```python
from build123d import *

# Parameters (mm, degrees)
SKETCH1_R           = 12.5
BOSS_EXTRUDE1_DEPTH = 2.5
SKETCH2_R           = 1.35
CUT_EXTRUDE1_DEPTH  = 18.853571071
SKETCH4_R           = 2.1
CUT_EXTRUDE2_DEPTH  = 1.5
CIRPATTERN1_COUNT   = 4
SKETCH3_R           = 1.35
BOSS_EXTRUDE2_DEPTH = 6
FILLET2_R           = 2
FILLET3_R           = 2


with BuildPart() as part:
    # Sketch1 → Boss-Extrude1 (new body)
    with BuildSketch(Plane(origin=(0, 0, 0), x_dir=(1, 0, 0), z_dir=(0, 1, 0))):
        with Locations(Location((0, 0, 0), (0, 0, 270))):
            Circle(SKETCH1_R)
    extrude(amount=BOSS_EXTRUDE1_DEPTH)

    # Sketch2 → Cut-Extrude1 (cut, through all)
    with BuildSketch(Plane(origin=(0, 2.5, 0), x_dir=(1, 0, 0), z_dir=(0, 1, 0))):
        with Locations(Location((0, 9.5, 0), (0, 0, 270))):
            Circle(SKETCH2_R)
    cut_extrude1 = extrude(amount=-CUT_EXTRUDE1_DEPTH, mode=Mode.SUBTRACT)

    # Sketch4 → Cut-Extrude2 (cut)
    with BuildSketch(Plane(origin=(0, 2.5, 0), x_dir=(1, 0, 0), z_dir=(0, 1, 0))):
        with Locations(Location((0, 9.5, 0), (0, 0, 270))):
            Circle(SKETCH4_R)
    cut_extrude2 = extrude(amount=-CUT_EXTRUDE2_DEPTH, mode=Mode.SUBTRACT)

    # CirPattern1: Cut-Extrude1, Cut-Extrude2 ×4 about axis
    cirpattern1_axis = Axis((0, 0, 0), (0, 1, 0))
    add([cut_extrude1.rotate(cirpattern1_axis, i * 360 / CIRPATTERN1_COUNT) for i in range(1, CIRPATTERN1_COUNT)], mode=Mode.SUBTRACT)
    add([cut_extrude2.rotate(cirpattern1_axis, i * 360 / CIRPATTERN1_COUNT) for i in range(1, CIRPATTERN1_COUNT)], mode=Mode.SUBTRACT)

    # Sketch3 → Boss-Extrude2 (add)
    with BuildSketch(Plane(origin=(0, 2.5, 0), x_dir=(1, 0, 0), z_dir=(0, 1, 0))):
        with Locations(Location((0, 0, 0), (0, 0, 270))):
            Circle(SKETCH3_R)
    extrude(amount=BOSS_EXTRUDE2_DEPTH)

    # Fillet2
    fillet2_edges = [part.edges().sort_by_distance(p)[0] for p in [
        (0, 2.5, -1.35),
    ]]
    fillet(fillet2_edges, radius=FILLET2_R)

    # Fillet3
    # the kernel refuses this fillet: 2 mm, written as the material it takes off along each edge
    with BuildSketch(Plane(origin=(0, 2.5, 0), x_dir=(0, 0, 1), z_dir=(-1, 0, 0))) as fillet3_piece_1:
        with BuildLine():
            CenterArc((12.5 - FILLET3_R, -FILLET3_R), FILLET3_R, 0, 90)
            Line((12.5, -FILLET3_R), (12.5, 0))
            Line((12.5, 0), (12.5 - FILLET3_R, 0))
        make_face()
    revolve(axis=Axis((0, 2.5, 0), (0, 1, 0)), mode=Mode.SUBTRACT)


solid = part.part
```
Here's how the part is built. I have some questions about the finished solid (model axes, mm). A direction names the side the tool comes from. Give positions to 0.01 mm unless a question says otherwise; leave off trailing zeros. Loops run counter-clockwise (first coordinate to the right, second up) from the corner with the lowest first, then second, coordinate; pieces in that order, holes last. Notation, with made-up numbers: (68, 74) -> (85, 74) arc R26 ccw to (85, 111) -> close; hole circle Ø10 at (-8, 33). An arc over 180 degrees is marked (long way). Use one line per item in the form item = value. Start each with the question number.
1) Imagine slicing it at B-B (y = 5). Please give me the cut outline in (x, z), then the cut area to 3 significant figures.
2) Please list where these lines run through material, in increasing order: line 1 along Y through (x, z) = (-7, -6.25); line 2 along X through (y, z) = (1.75, -9.75); line 3 along Z through (x, y) = (-8, 1.75).
3) Thinking about a two-plate mould opening in Z: for faces 3 (the face through (-8, 1, 0)), 4 (the face through (0, 2.5, -5)), 5 (the face through (3.755, 0.246, 11.923)), which applies, +Z half, -Z half, draft (parallel to the pull), parting line (faces both ways), or undercut?
4) Which directions (+Z, -Z, +X, -X, +Y, -Y) give clear straight access to the entire face, cutting with the end or side of a thin tool? Please do faces 1 (the face through (8.212, 0.507, 0.406)), 2 (the face through (-7.497, 1.76, -0.631)).
5) For P1, Ø6, axis at x = -3, z = -3.5, coming from the +Y side; P2, Ø3.5, axis at x = -9.5, z = 0, coming from the +Y side; P3, Ø2, axis at y = 4.5, z = -7.5, coming from the +X side; P4, Ø3, axis at x = 3, z = -4.5, coming from the +Y side, each with a flat end and sliding along its axis, tell me the tip position at first contact or that it passes through.
6) Imagine slicing it at A-A (z = 0). Please give me the cut outline in (x, y).
Check values:
q1.outline = circle Ø2.7 at (0, 0)
q1.area = 5.73 mm^2
q2.line_1 = 0 to 2.5
q2.line_2 = -7.1 to -2.09, 2.09 to 7.1
q2.line_3 = -9.03 to -1.47, 1.47 to 9.03
q3.face_3 = undercut
q3.face_4 = draft
q3.face_5 = parting line
q4.face_1 = +Y, -Y
q4.face_2 = +Y
q5.P1 = 3.51
q5.P2 = 1
q5.P3 = through
q5.P4 = 2.5
q6.outline = (-12.5, 0) -> (-10.85, 0) -> (-10.85, 1) -> (-11.6, 1) -> (-11.6, 2.17) arc R2 ccw to (-12.5, 0.5) -> close; (-8.15, 0) -> (8.15, 0) -> (8.15, 1) -> (7.4, 1) -> (7.4, 2.5) -> (3.35, 2.5) arc R2 cw to (1.35, 4.5) -> (1.35, 8.5) -> (-1.35, 8.5) -> (-1.35, 4.5) arc R2 cw to (-3.35, 2.5) -> (-7.4, 2.5) -> (-7.4, 1) -> (-8.15, 1) -> close; (10.85, 0) -> (12.5, 0) -> (12.5, 0.5) arc R2 ccw to (11.6, 2.17) -> (11.6, 1) -> (10.85, 1) -> close
